Autodesk Fusion 360 part; units mm, degrees
sketch "Sketch1" plane through (0, 0, 0) normal (0, 1, 0) x (1, 0, 0)
  line L0 (40, -40) -> (-40, -40)
  line L1 (-40, -40) -> (-40, 40)
  line L2 (-40, 40) -> (40, 40)
  line L3 (40, 40) -> (40, -40)
  line L4 (40, -40) -> (-40, 40) construction
  line L5 (-40, -40) -> (40, 40) construction
  dimension "d1" = 80
  dimension "d2" = 80
extrude "Extrude1" add sketch "Sketch1" along normal blind 20
sketch "Sketch2" plane through (0, 20, 0) normal (0, 1, 0) x (-1, 0, 0)
  line L0 (-40, -40) -> (40, -40)
  line L1 (40, -40) -> (40, 40)
  line L2 (40, 40) -> (-40, 40)
  line L3 (-40, 40) -> (-40, -40)
  line L4 (40, -40) -> (35, -40)
  line L5 (-40, -40) -> (-35, -40)
  line L6 (40, -40) -> (40, -35)
  line L7 (-40, -40) -> (-40, -35)
  line L8 (40, 40) -> (40, 35)
  line L9 (40, 40) -> (35, 40)
  line L10 (-40, 40) -> (-40, 35)
  line L11 (-40, 40) -> (-35, 40)
  circle A0 centre (35, 35) radius 3.75
  circle A1 centre (-35, 35) radius 3.75
  circle A2 centre (35, -35) radius 3.75
  circle A3 centre (-35, -35) radius 3.75
  line L12 (-30, 30) -> (30, 30)
  line L13 (30, 30) -> (30, -30)
  line L14 (30, -30) -> (-30, -30)
  line L15 (-30, -30) -> (-30, 30)
  line L16 (-30, 30) -> (30, -30) construction
  line L17 (30, 30) -> (-30, -30) construction
  dimension "d5" = 5
  dimension "d6" = 5
  dimension "d7" = 5
  dimension "d8" = 5
  dimension "d9" = 5
  dimension "d10" = 5
  dimension "d11" = 5
  dimension "d12" = 5
  dimension "d13" = 7.5
  dimension "d14" = 7.5
  dimension "d15" = 7.5
  dimension "d16" = 7.5
  dimension "d25" = 60
  dimension "d26" = 60
extrude "Extrude6" cut sketch "Sketch2" against normal blind 8.5 contours L12 L13 L14 L15
extrude "Extrude2" cut sketch "Sketch2" against normal blind 5 contours A0
extrude "Extrude3" cut sketch "Sketch2" against normal blind 5 contours A2
extrude "Extrude4" cut sketch "Sketch2" against normal blind 5 contours A1
extrude "Extrude5" cut sketch "Sketch2" against normal blind 5 contours A3
thread "Thread1"
thread "Thread2"
thread "Thread3"
thread "Thread4"
fillet "Fillet1" radius 0.5 1 edges at (40, 10, 40)
fillet "Fillet2" radius 0.5 1 edges at (-40, 10, 40)
fillet "Fillet3" radius 0.5 1 edges at (40, 10, -40)
fillet "Fillet4" radius 0.5 1 edges at (-40, 10, -40)
Input: part model. Units: mm. Frame: model coordinates. A direction names the side the tool comes from. Round coordinates to 2 decimals unless told otherwise and drop trailing zeros. Loops run counter-clockwise (first coordinate to the right, second up) from the corner with the lowest first, then second, coordinate; pieces in that order, holes last. Notation, with made-up numbers: M 40.25,-31.75 L 74.25,-31.75 A14 ccw 74.25,-17.75 Z; hole C -3,57 d9. An arc over 180 degrees is marked long. Answer as CSV lines item,"result". Start each with the question number.
(1) First-contact query: pin 1 (2 mm diameter, centred on x = -34, z = 36.5, fed in from +Y); pin 2 (8 mm diameter, centred on x = -21, z = -21, fed in from +Y). Flat tips, straight axial feed; report the tip coordinate or a pass-through.
(2) Section C-C, the plane x = 4.5. Output: boundary loops of the cut face in (y, z).
(3) Draft query along Z for faces 3 (the flat face through (-1, 0, -1)), 4 (the flat face through (-35, 15, 35)), 5 (the flat face through (1, 10, 40)). Return one class per face: released by +Z, released by -Z, zero draft, split by the parting line, or undercut.
(4) Section A-A, the plane x = 35. Output: boundary loops of the cut face in (y, z).
(5) Section B-B, the plane z = -35. Output: boundary loops of the cut face in (x, y), plus the area to 4 significant figures.
(6) Section D-D, the plane z = -24. Output: boundary loops of the cut face in (x, y).
(7) Reachability of faces 1 (the flat face through (-40, 10, 1)), 2 (the cylindrical face through (38.746, 17.535, -34.835)) from +Z, -Z, +X, -X, +Y, -Y: full face, straight path, thin tool, end or side. Return the list, or none.
(8) Line query: line 1 (Z direction, x = -35, y = 16.7); line 2 (X direction, y = 15.5, z = -12.5). Output: solid intervals per line, ascending. Write a range as [from, to].
Values found:
1,pin 1,"stops at y = 15"
1,pin 2,"stops at y = 11.5"
2,outline,"M 0,-40 L 20,-40 L 20,-30 L 11.5,-30 L 11.5,30 L 20,30 L 20,40 L 0,40 Z"
3,face 3,"zero draft"
3,face 4,"undercut"
3,face 5,"released by +Z"
4,outline,"M 0,-40 L 20,-40 L 20,-38.75 L 15,-38.75 L 15,-31.25 L 20,-31.25 L 20,31.25 L 15,31.25 L 15,38.75 L 20,38.75 L 20,40 L 0,40 Z"
5,outline,"M -40,0 L 40,0 L 40,20 L 38.75,20 L 38.75,15 L 31.25,15 L 31.25,20 L -31.25,20 L -31.25,15 L -38.75,15 L -38.75,20 L -40,20 Z"
5,area,"1,525 mm²"
6,outline,"M -40,0 L 40,0 L 40,20 L 30,20 L 30,11.5 L -30,11.5 L -30,20 L -40,20 Z"
7,face 1,"+Z, -Z, -X, +Y, -Y"
7,face 2,"+Y"
8,line 1,"z = [-40, -38.75], [-31.25, 31.25], [38.75, 40]"
8,line 2,"x = [-40, -30], [30, 40]"
